Geometry: see drawing. Coordinates: mm, zero at the bounding-box minimum. Give positions to 0.01 mm unless a question says otherwise; leave off trailing zeros. Write each loop counter-clockwise with the first axis right and the second up, starting at its lowest first coordinate (ties: lowest second). Pieces come first, ordered by that corner, then holes. Notation, with made-up numbers: (-9.75, 33.25) -> (2.25, 33.25) arc R25 ccw to (2.25, 72.25) -> close; hole circle Ø3 at (43.25, 8.25). An arc over 180 degrees is marked (long way). Answer as a JSON object with one key per item and string values. Group by question number.
Item 1: Section query D-D on x = 195. Return the cut outline in (y, z), plus the area to 3 significant figures.
Item 2: Ray query, probe 1 along Y at (x, z) = (360, 1.4); probe 2 along Y at (x, z) = (263.5, 2.3); probe 3 along Y at (x, z) = (67, 0.95). Return the intervals inside material, ascending. Write a range as from..to.
Item 3: Section query C-C on y = 33. Return the cut outline in (x, z).
Item 4: Section query B-B on z = 0.95. Give the number of separate pieces and of enclosed holes in the cut face, plus the area to 3 significant figures.
Item 5: Section query A-A on x = 360. Return the cut outline in (y, z), plus the area to 3 significant figures.
Item 6: First-contact query: pin 1 Ø1 at (x, z) = (82.5, 2) entering from -Y; pin 2 Ø1.5 at (y, z) = (1, 2) entering from -X. Flat tips, straight axial feed; report the tip coordinate or a pass-through.
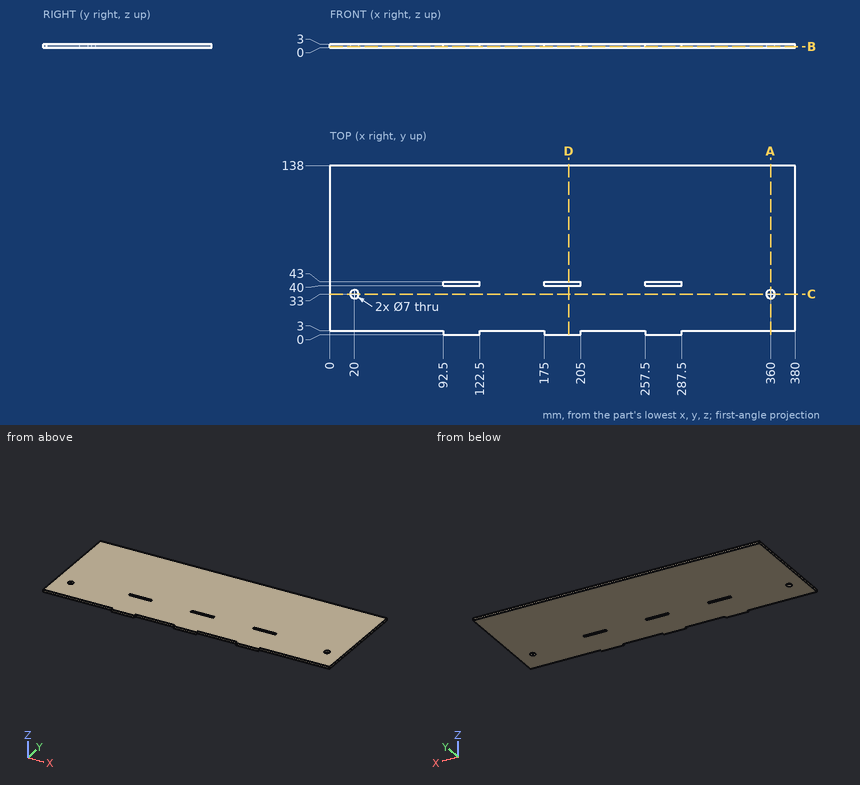
Worked answers:
{
 "1": {"outline": "(0, 0) -> (40, 0) -> (40, 3) -> (0, 3) -> close; (43, 0) -> (138, 0) -> (138, 3) -> (43, 3) -> close", "area": "405 mm^2"},
 "2": {"probe 1": "3..29.5, 36.5..138", "probe 2": "0..40, 43..138", "probe 3": "3..138"},
 "3": {"outline": "(0, 0) -> (16.5, 0) -> (16.5, 3) -> (0, 3) -> close; (23.5, 0) -> (356.5, 0) -> (356.5, 3) -> (23.5, 3) -> close; (363.5, 0) -> (380, 0) -> (380, 3) -> (363.5, 3) -> close"},
 "4": {"separate pieces": "1", "enclosed holes": "5", "area": "51,200 mm^2"},
 "5": {"outline": "(3, 0) -> (29.5, 0) -> (29.5, 3) -> (3, 3) -> close; (36.5, 0) -> (138, 0) -> (138, 3) -> (36.5, 3) -> close", "area": "384 mm^2"},
 "6": {"pin 1": "y = 3", "pin 2": "x = 92.5"}
}
